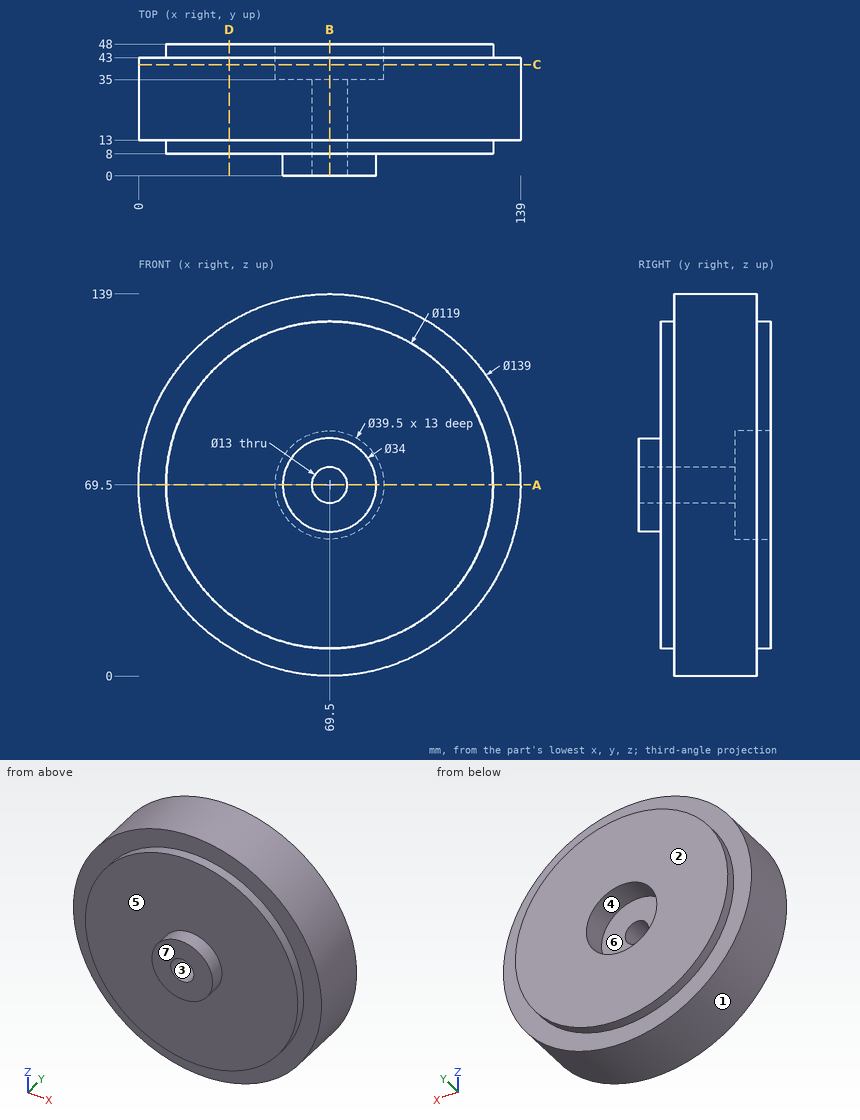
Job drawing, mm, ordinate dimensions from the low corner. One solid piece. A direction names the side the tool comes from. Round coordinates to 2 decimals unless told otherwise and drop trailing zeros. Loops run counter-clockwise (first coordinate to the right, second up) from the corner with the lowest first, then second, coordinate; pieces in that order, holes last.
Item 1: Mould opens along Z. For the marked faces 1, 2, 3 and 4 say: +Z half, -Z half, draft (parallel to the pull), parting line (faces both ways), or undercut.
Item 2: Drop flat-ended pins along their axis: P1, Ø17, axis at x = 69.5, z = 69.5, coming from the +Y side; P2, Ø2, axis at x = 28, y = 15, coming from the +Z side; P3, Ø6, axis at y = 30.5, z = 90, coming from the +X side. Give the stop position or say it passes through.
Item 3: Cut at C-C, the plane y = 40.5. Give the cut face in (x, z).
Item 4: Cut at A-A, the plane z = 69.5. Give the cut face in (x, y), then the cut area to 3 significant figures.
Item 5: Cut at B-B, the plane x = 69.5. Give the cut face in (y, z).
Item 6: Drill centre lines: line 1 (X direction, y = 39, z = 69.5); line 2 (X direction, y = 17, z = 69.5); line 3 (Y direction, x = 65, z = 33). Where is each one in solid material? Low to high.
Item 7: 3-axis set-ups, long thin cutter, end or side, ignore diameter. For the marked faces 5, 6 and 7: which of +Z, -Z, +X, -X, +Y, -Y reach the whole face in a straight line?
Item 8: Cut at D-D, the plane x = 33. Give the cut face in (y, z).
A:
1. face 1: parting line
1. face 2: draft
1. face 3: undercut
1. face 4: undercut
2. P1: stops at y = 35
2. P2: stops at z = 125.98
2. P3: stops at x = 136.76
3. outline: circle Ø139 at (69.5, 69.5); hole circle Ø39.5 at (69.5, 69.5)
4. outline: (0, 13) - (10, 13) - (10, 8) - (52.5, 8) - (52.5, 0) - (63, 0) - (63, 35) - (49.75, 35) - (49.75, 48) - (10, 48) - (10, 43) - (0, 43) - close; (76, 0) - (86.5, 0) - (86.5, 8) - (129, 8) - (129, 13) - (139, 13) - (139, 43) - (129, 43) - (129, 48) - (89.25, 48) - (89.25, 35) - (76, 35) - close
4. area: 4,660 mm2
5. outline: (0, 52.5) - (8, 52.5) - (8, 10) - (13, 10) - (13, 0) - (43, 0) - (43, 10) - (48, 10) - (48, 49.75) - (35, 49.75) - (35, 63) - (0, 63) - close; (0, 76) - (35, 76) - (35, 89.25) - (48, 89.25) - (48, 129) - (43, 129) - (43, 139) - (13, 139) - (13, 129) - (8, 129) - (8, 86.5) - (0, 86.5) - close
6. line 1: x = 0 to 49.75, 89.25 to 139
6. line 2: x = 0 to 63, 76 to 139
6. line 3: y = 8 to 48
7. face 5: -Y
7. face 6: +Y
7. face 7: +Z, -Z, +X, -X, -Y
8. outline: (8, 22.51) - (13, 22.51) - (13, 10.36) - (43, 10.36) - (43, 22.51) - (48, 22.51) - (48, 116.49) - (43, 116.49) - (43, 128.64) - (13, 128.64) - (13, 116.49) - (8, 116.49) - close
